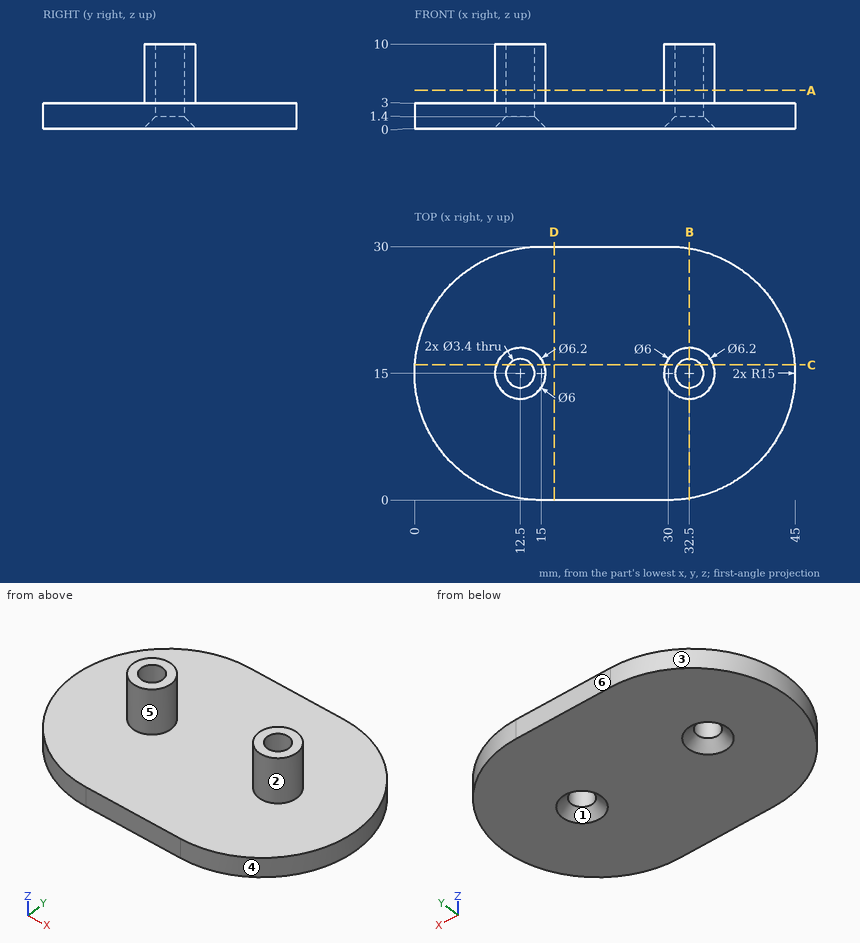
The figure shows three views and two pictorial views of one solid part (mm, origin at its lowest corner). Answer the questions. A direction names the side the tool comes from. Round coordinates to 2 decimals unless told otherwise and drop trailing zeros. Write each loop counter-clockwise with the first axis right and the second up, starting at its lowest first coordinate (ties: lowest second). Pieces come first, ordered by that corner, then holes. Notation, with made-up numbers: M -28.5,87 L 11.5,87 A27 cw 11.5,120 Z; hole C 26,67 d11. An arc over 180 degrees is marked long. Use a Markdown table: item, result.
1) The part is cut by section A-A (z = 4.5). Write down the section's boundary in (x, y).
Answers follow:
| item | result |
|---|---|
| outline | C 12.5,15 d6; C 32.5,15 d6; hole C 12.5,15 d3.4; hole C 32.5,15 d3.4 |
2) The part is cut by section B-B (x = 32.5). Write down the section's boundary in (y, z).
Answers follow:
| item | result |
|---|---|
| outline | M 0.21,0 L 11.9,0 L 13.3,1.4 L 13.3,10 L 12,10 L 12,3 L 0.21,3 Z; M 16.7,1.4 L 18.1,0 L 29.79,0 L 29.79,3 L 18,3 L 18,10 L 16.7,10 Z |
3) The part is cut by section C-C (y = 16). Give the number of separate pieces and of enclosed holes in the cut face, plus the area to 3 significant figures.
Answers follow:
| item | result |
|---|---|
| separate pieces | 3 |
| enclosed holes | 0 |
| area | 155 mm2 |
4) The part is cut by section D-D (x = 16.5). Write down the section's boundary in (y, z), plus the area to 3 significant figures.
Answers follow:
| item | result |
|---|---|
| outline | M 0,0 L 30,0 L 30,3 L 0,3 Z |
| area | 90.0 mm2 |
5) For a pull along X with two mould halves and no side action, classify the marked faces 3, 4, 5 and 6 as pulls with the +X half, pulls with the -X half, needs draft (parallel to the pull), parting line crosses it, or undercut.
Answers follow:
| item | result |
|---|---|
| face 3 | pulls with the -X half |
| face 4 | pulls with the +X half |
| face 5 | undercut |
| face 6 | needs draft |
6) Straight lines are drawn through the part: line 1 along X through (y, z) = (13.5, 3.25); line 2 along Y through (x, z) = (12.5, 8.25); line 3 along Z through (x, y) = (3, 11). For each, find the intervals that lie inside material, in ascending order. Write a range as [from, to].
Answers follow:
| item | result |
|---|---|
| line 1 | x = [9.9, 11.7], [13.3, 15.1], [29.9, 31.7], [33.3, 35.1] |
| line 2 | y = [12, 13.3], [16.7, 18] |
| line 3 | z = [0, 3] |
7) Flat-ended cylindrical pins translate along their axes: pin 1 (8 mm diameter, centred on x = 10.5, y = 25.5, fed in from +Z); pin 2 (1 mm diameter, centred on x = 12, y = 4, fed in from -Z); pin 3 (3 mm diameter, centred on y = 8.5, z = 2, fed in from +X). Find the tip coordinate at first contact, or state that the pin passes through.
Answers follow:
| item | result |
|---|---|
| pin 1 | stops at z = 3 |
| pin 2 | stops at z = 0 |
| pin 3 | stops at x = 44.14 |
8) A tool of negligible diameter and unlimited length cuts with its end or side. For the marked faces 1 and 2, from which of +Z, -Z, +X, -X, +Y, -Y can it reach the whole face along a straight path? Write none if from no direction.
Answers follow:
| item | result |
|---|---|
| face 1 | -Z |
| face 2 | +Z |
